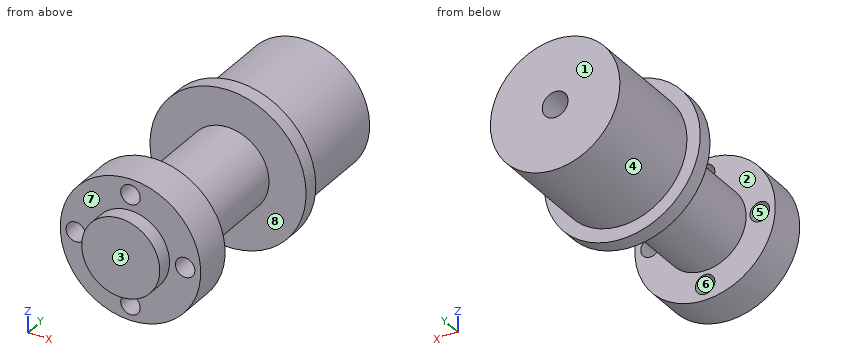
```python
from build123d import *

# Parameters (mm, degrees)
SKETCH_1_R             = 9
EXTRUDE_1_DEPTH        = 5
SKETCH_3_R             = 5.25
EXTRUDE_2_DEPTH        = 15
SKETCH_4_R             = 10
EXTRUDE_4_DEPTH        = 2
SKETCH_5_R             = 8.3
EXTRUDE_5_DEPTH        = 13.75
HOLE_WIZARD_M3_1_D     = 2.5
HOLE_WIZARD_M3_1_DEPTH = 5
SKETCH_8_R             = 5
EXTRUDE_6_DEPTH        = 2
HOLE_WIZARD_M4_3_D     = 3.3
HOLE_WIZARD_M4_3_DEPTH = 10.1
HOLE_WIZARD_M4_3_TIP   = 0.991420021


with BuildPart() as part:
    # 草图1 → 凸台-拉伸1 (new body)
    with BuildSketch(Plane(origin=(0, 0, 0), x_dir=(1, 0, 0), z_dir=(0, 1, 0))):
        with Locations(Location((0, 0, 0), (0, 0, 270))):
            Circle(SKETCH_1_R)
    extrude(amount=EXTRUDE_1_DEPTH)

    # 草图3 → 凸台-拉伸2 (add)
    with BuildSketch(Plane(origin=(0, 5, 0), x_dir=(1, 0, 0), z_dir=(0, 1, 0))):
        with Locations(Location((0, 0, 0), (0, 0, 270))):
            Circle(SKETCH_3_R)
    extrude(amount=EXTRUDE_2_DEPTH)

    # 草图4 → 凸台-拉伸4 (add)
    with BuildSketch(Plane(origin=(0, 20, 0), x_dir=(1, 0, 0), z_dir=(0, 1, 0))):
        with Locations(Location((0, 0, 0), (0, 0, 270))):
            Circle(SKETCH_4_R)
    extrude(amount=EXTRUDE_4_DEPTH)

    # 草图5 → 凸台-拉伸5 (add)
    with BuildSketch(Plane(origin=(0, 22, 0), x_dir=(1, 0, 0), z_dir=(0, 1, 0))):
        with Locations(Location((0, 0, 0), (0, 0, 270))):
            Circle(SKETCH_5_R)
    extrude(amount=EXTRUDE_5_DEPTH)

    # M3 螺纹孔1
    with Locations(Plane(origin=(0, 0, 0), x_dir=(-1, 0, 0), z_dir=(0, -1, 0))):
        with Locations((0, 7), (-7, 0), (7, 0), (0, -7)):
            Hole(HOLE_WIZARD_M3_1_D / 2, depth=HOLE_WIZARD_M3_1_DEPTH)

    # 草图8 → 凸台-拉伸6 (add)
    with BuildSketch(Plane.XZ):
        with Locations(Location((0, 0, 0), (0, 0, 270))):
            Circle(SKETCH_8_R)
    extrude(amount=EXTRUDE_6_DEPTH)

    # M4 螺纹孔3
    with Locations(Plane(origin=(0, 35.75, 0), x_dir=(1, 0, 0), z_dir=(0, 1, 0))):
        with Locations((0, 0)):
            Hole(HOLE_WIZARD_M4_3_D / 2, depth=HOLE_WIZARD_M4_3_DEPTH)
            with Locations((0, 0, -(HOLE_WIZARD_M4_3_DEPTH + HOLE_WIZARD_M4_3_TIP / 2))):  # 118° drill point
                Cone(0, HOLE_WIZARD_M4_3_D / 2, HOLE_WIZARD_M4_3_TIP, mode=Mode.SUBTRACT)


solid = part.part
```
Check sheet for the modelled part. Datum: model origin and axes. Units: mm. Face numbers are marked on the shaded views. A direction names the side the tool comes from. Give positions to 0.01 mm unless a question says otherwise; leave off trailing zeros. Order: outer loops, then holes, each group sorted by start corner. A loop starts at its lowest first (then second) coordinate and runs counter-clockwise, first axis right, second up. Notation, with made-up numbers: (-5, -18) -> (51, -18) arc R15 cw to (51, 10) -> close; hole circle Ø5 at (-10, -8). An arc over 180 degrees is marked (long way). Return JSON: item names as keys, results as strings.
1. Mould release check, pull along Y, two halves, no side actions. Record for the marked faces 6, 7 and 8: +Y half, -Y half, draft (parallel to the pull), parting line (faces both ways), or undercut.
From the geometry:
{"face 6": "draft", "face 7": "-Y half", "face 8": "undercut"}
2. Cross-section at C-C, the plane y = 11.5. Record the cut outline in (x, z).
From the geometry:
{"outline": "circle Ø10.5 at (0, 0)"}
3. Set-up check for the marked faces 1, 2, 3, 4 and 5: record each of +Z, -Z, +X, -X, +Y, -Y from which the full face is reachable in a straight line by a thin tool's end or side.
From the geometry:
{"face 1": "+Z, -Z, +X, -X, +Y", "face 2": "none", "face 3": "+Z, -Z, +X, -X, -Y", "face 4": "+Y", "face 5": "-Y"}
4. Cross-section at D-D, the plane x = -2.5. Record the cut outline in (y, z).
From the geometry:
{"outline": "(-2, -4.33) -> (0, -4.33) -> (0, -8.65) -> (5, -8.65) -> (5, -4.62) -> (20, -4.62) -> (20, -9.68) -> (22, -9.68) -> (22, -7.91) -> (35.75, -7.91) -> (35.75, 7.91) -> (22, 7.91) -> (22, 9.68) -> (20, 9.68) -> (20, 4.62) -> (5, 4.62) -> (5, 8.65) -> (0, 8.65) -> (0, 4.33) -> (-2, 4.33) -> close"}
5. Go/stop test with flat-tipped pins: P1, Ø3, axis at x = -2.5, y = 4, coming from the -Z side; P2, Ø3, axis at x = 0, z = -7, coming from the -Y side; P3, Ø2, axis at x = -4.5, y = 24, coming from the +Z side; P4, Ø9, axis at x = -1, z = 0.5, coming from the +Y side. Record where each tip stops, or that it passes through.
From the geometry:
{"P1": "z = -8.94", "P2": "y = 0", "P3": "z = 7.53", "P4": "y = 35.75"}
6. Cross-section at B-B, the plane z = 7. Record the cut outline in (x, y).
From the geometry:
{"outline": "(-7.14, 20) -> (7.14, 20) -> (7.14, 22) -> (4.46, 22) -> (4.46, 35.75) -> (-4.46, 35.75) -> (-4.46, 22) -> (-7.14, 22) -> close; (-5.66, 0) -> (-1.25, 0) -> (-1.25, 5) -> (-5.66, 5) -> close; (1.25, 0) -> (5.66, 0) -> (5.66, 5) -> (1.25, 5) -> close"}
7. Cross-section at A-A, the plane x = -6.25. Record the cut outline in (y, z), plus the area to 3 significant figures.
From the geometry:
{"outline": "(0, -6.48) -> (5, -6.48) -> (5, -1) -> (0, -1) -> close; (0, 1) -> (5, 1) -> (5, 6.48) -> (0, 6.48) -> close; (20, -7.81) -> (22, -7.81) -> (22, -5.46) -> (35.75, -5.46) -> (35.75, 5.46) -> (22, 5.46) -> (22, 7.81) -> (20, 7.81) -> close", "area": "236 mm^2"}
8. Material ranges on probe 1 along Y at (x, z) = (5.5, -3.25); probe 2 along Y at (x, z) = (7, -5); probe 3 along Y at (x, z) = (9, 3), recorded low to high. Write a range as [from, to].
From the geometry:
{"probe 1": "[0, 5], [20, 35.75]", "probe 2": "[0, 5], [20, 22]", "probe 3": "[20, 22]"}
